```python
from build123d import *

# Parameters (mm, degrees)
SKETCH18_W          = 200
SKETCH18_H          = 23.014216905
BOSS_EXTRUDE4_DEPTH = 1.5
BOSS_EXTRUDE5_DEPTH = 1.5


with BuildPart() as part:
    # Sketch18 → Boss-Extrude4 (new body)
    with BuildSketch(Plane.XY):
        with Locations((39.219715871, 11.507108453)):
            Rectangle(SKETCH18_W, SKETCH18_H)
    extrude(amount=BOSS_EXTRUDE4_DEPTH)

    # Sketch16 → Boss-Extrude5 (add)
    with BuildSketch(Plane(origin=(0, 0, 0), x_dir=(1, 0, 0), z_dir=(0, 1, 0))):
        Polygon((-47.784100803, 22.510049826), (126.22317902, 22.510049826), (139.219715871, 0), (-60.780284129, 0), align=None)
    extrude(amount=BOSS_EXTRUDE5_DEPTH)


solid = part.part
```
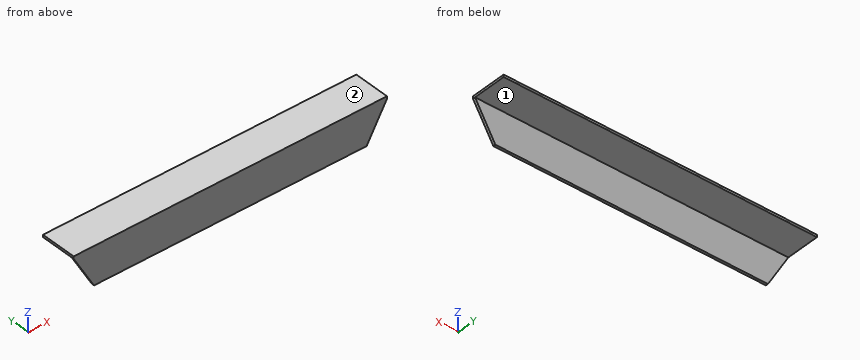
Source: CAD feature listing. Evaluate the final solid. Frame: model axes, mm. Face numbers are marked on the shaded views. A direction names the side the tool comes from. Coordinates: 2 decimals unless noted, no trailing zeros. Loops run counter-clockwise (first coordinate to the right, second up) from the corner with the lowest first, then second, coordinate; pieces in that order, holes last. Notation, with made-up numbers: M 0.25,74 L 25.25,74 A19 cw 25.25,79 Z; hole C 48,31.25 d10. An arc over 180 degrees is marked long. Use CSV: the item, a comma, the result in double quotes.
(1) Reachability of the marked faces 1 and 2 from +Z, -Z, +X, -X, +Y, -Y: full face, straight path, thin tool, end or side. Return the list, or none.
Answers follow:
face 1,"-Z, +X, -X, +Y"
face 2,"+Z, +X, -X, +Y, -Y"
(2) Cut plane A-A on x = 96.5. Return loops of the section in (y, z).
Answers follow:
outline,"M 0,-22.51 L 1.5,-22.51 L 1.5,0 L 23.01,0 L 23.01,1.5 L 0,1.5 Z"
(3) Cut plane C-C on z = -15.5. Return loops of the section in (x, y).
Answers follow:
outline,"M -51.83,0 L 130.27,0 L 130.27,1.5 L -51.83,1.5 Z"
(4) Cut plane B-B on y = 20.25. Return loops of the section in (x, z).
Answers follow:
outline,"M -60.78,0 L 139.22,0 L 139.22,1.5 L -60.78,1.5 Z"
(5) Line query: line 1 (Z direction, x = 125, y = 7.25). Output: solid intervals per line, ascending. Write a range as [from, to].
Answers follow:
line 1,"[0, 1.5]"
